Design review of the part built by this model. Coordinates are the model's own, in mm. Face numbers are marked on the shaded views. A direction names the side the tool comes from. Give positions to 0.01 mm unless a question says otherwise; leave off trailing zeros. Loops run counter-clockwise (first coordinate to the right, second up) from the corner with the lowest first, then second, coordinate; pieces in that order, holes last. Notation, with made-up numbers: (1, 44.25) - (27, 44.25) arc R12 cw to (27, 58.25) - close; hole circle Ø8 at (-5, -20.5). An arc over 180 degrees is marked (long way). Write each question's results on one line, items separated by ' | '.
Autodesk Inventor part; units mm, degrees
ref_plane "Work Plane1" through (2, 0, 0) normal (1, 0, 0) x (0, 0, -1)
ref_plane "YZ Plane" through (0, 0, 0) normal (1, 0, 0) x (0, 1, 0)
ref_plane "XZ Plane" through (0, 0, 0) normal (0, 1, 0) x (-1, 0, 0)
sketch "Sketch1" plane through (0, 0, 0) normal (1, 0, 0) x (0, 1, 0)
  circle A0 centre (0, 0) radius 1.5
  dimension "d0" = 3
extrude "Extrusion1" add sketch "Sketch1" against normal blind 5.5
ref_plane "Work Plane1" through (2, 0, 0) normal (1, 0, 0) x (0, 0, -1)
sketch "Sketch2" plane through (2, 0, 0) normal (1, 0, 0) x (0, 0, -1)
  circle A0 centre (0, 0) radius 3.75
  dimension "d4" = 7.5
loft "Loft1" add profiles "Sketch2" section 1 edges at (0, -1.5, 0)
sketch "Sketch3" plane through (2, 0, 0) normal (1, 0, 0) x (0, 0, -1)
  line L0 (-0.5, -1.75) -> (0.5, -1.75)
  line L1 (0.5, 1.75) -> (-0.5, 1.75)
  line L2 (1.75, -0.5) -> (1.75, 0.5)
  line L3 (-1.75, 0.5) -> (-1.75, -0.5)
  line L4 (0.5, -1.75) -> (0.5, -0.866)
  line L5 (0.5, 0.866) -> (0.5, 1.75)
  line L6 (-1.75, -0.5) -> (-0.866, -0.5)
  line L7 (0.866, -0.5) -> (1.75, -0.5)
  arc A0 (0.5, -0.866) -> (0.866, -0.5) centre (0, 0) ccw
  line L8 (1.75, 0.5) -> (0.866, 0.5)
  line L9 (-0.866, 0.5) -> (-1.75, 0.5)
  line L10 (-0.5, 1.75) -> (-0.5, 0.866)
  line L11 (-0.5, -0.866) -> (-0.5, -1.75)
  arc A1 (0.866, 0.5) -> (0.5, 0.866) centre (0, 0) ccw
  arc A2 (-0.5, 0.866) -> (-0.866, 0.5) centre (0, 0) ccw
  arc A3 (-0.866, -0.5) -> (-0.5, -0.866) centre (0, 0) ccw
  dimension "d9" = 1
  dimension "d10" = 3.5
  dimension "d11" = 1
  dimension "d12" = 3.5
extrude "Extrusion2" cut sketch "Sketch3" against normal blind 1.5 draft -10
thread "Thread1"
properties part number "Parafuso do Escudo"
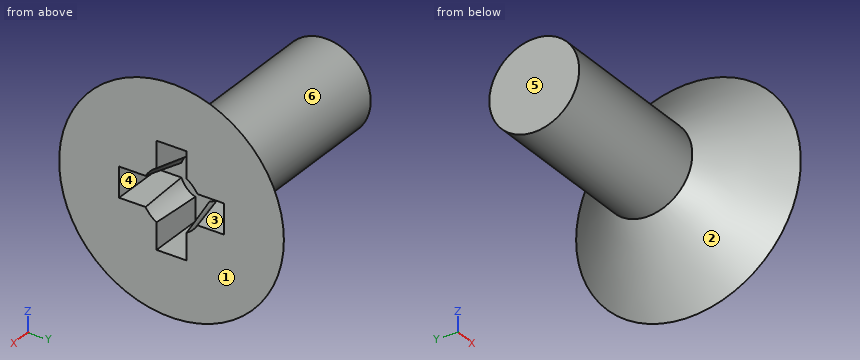
(1) Wall thickness on line 1 along Y through (x, z) = (1.75, 0.75); line 2 along Y through (x, z) = (1, -1.25); line 3 along Z through (x, y) = (1, 1.5): over which ranges is each line inside the solid? List them lowest first. Write a range as from..to.
Answers below:
line 1: -3.39..-0.59, 0.59..3.39 | line 2: -2.31..-0.32, 0.32..2.31 | line 3: -2.15..-0.32, 0.32..2.15
(2) Take a section at A-A on y = 0. Give the boundary of the cut face in (x, z).
Answers below:
outline: (-5.5, -1.5) - (0, -1.5) - (2, -3.75) - (2, -1.75) - (0.5, -1.49) - (0.5, 1.49) - (2, 1.75) - (2, 3.75) - (0, 1.5) - (-5.5, 1.5) - close
(3) Take a section at B-B on x = 1. Give the boundary of the cut face in (y, z) (3 decimals), plus the area to 3 significant figures.
Answers below:
outline: circle Ø5.25 at (0, 0); hole (-1.574, -0.324) - (-0.757, -0.324) arc R0.824 ccw to (-0.324, -0.757) - (-0.324, -1.574) - (0.324, -1.574) - (0.324, -0.757) arc R0.824 ccw to (0.757, -0.324) - (1.574, -0.324) - (1.574, 0.324) - (0.757, 0.324) arc R0.824 ccw to (0.324, 0.757) - (0.324, 1.574) - (-0.324, 1.574) - (-0.324, 0.757) arc R0.824 ccw to (-0.757, 0.324) - (-1.574, 0.324) - close | area: 17.5 mm2
(4) Draft analysis for pull direction Y (two halves, no side actions). For the marked faces 1, 2 and 3, state which applies: pulls with the +Y half, pulls with the -Y half, needs draft (parallel to the pull), parting line crosses it, or undercut.
Answers below:
face 1: needs draft | face 2: parting line crosses it | face 3: undercut
(5) Tool access review of the marked faces 4, 5 and 6: name each direction out of +Z, -Z, +X, -X, +Y, -Y from which nothing blocks a thin tool from reaching the whole face with its end or side.
Answers below:
face 4: +X | face 5: +Z, -Z, -X, +Y, -Y | face 6: -X
(6) Take a section at C-C on x = -2. Give the boundary of the cut face in (y, z), plus the area to 3 significant figures.
Answers below:
outline: circle Ø3 at (0, 0) | area: 7.07 mm2
(7) Insertion check: P1, Ø2, axis at x = 0, y = -0.5, coming from the +Z side; P2, Ø1, axis at x = -3, z = 0.5, coming from the -Y side; P3, Ø3, axis at x = -0.5, y = 2, coming from the -Z side; P4, Ø1.5, axis at y = -0.5, z = -0.5, coming from the +X side. Each pin has a flat end and moves straight along its axis. Give the tip position at first contact, or say it passes through.
Answers below:
P1: z = 2.59 | P2: y = -1.5 | P3: z = -2.05 | P4: x = 2
